Job drawing, mm, ordinate dimensions from the low corner. One solid piece. A direction names the side the tool comes from. Give positions to 0.01 mm unless a question says otherwise; leave off trailing zeros. Order: outer loops, then holes, each group sorted by start corner. A loop starts at its lowest first (then second) coordinate and runs counter-clockwise, first axis right, second up.
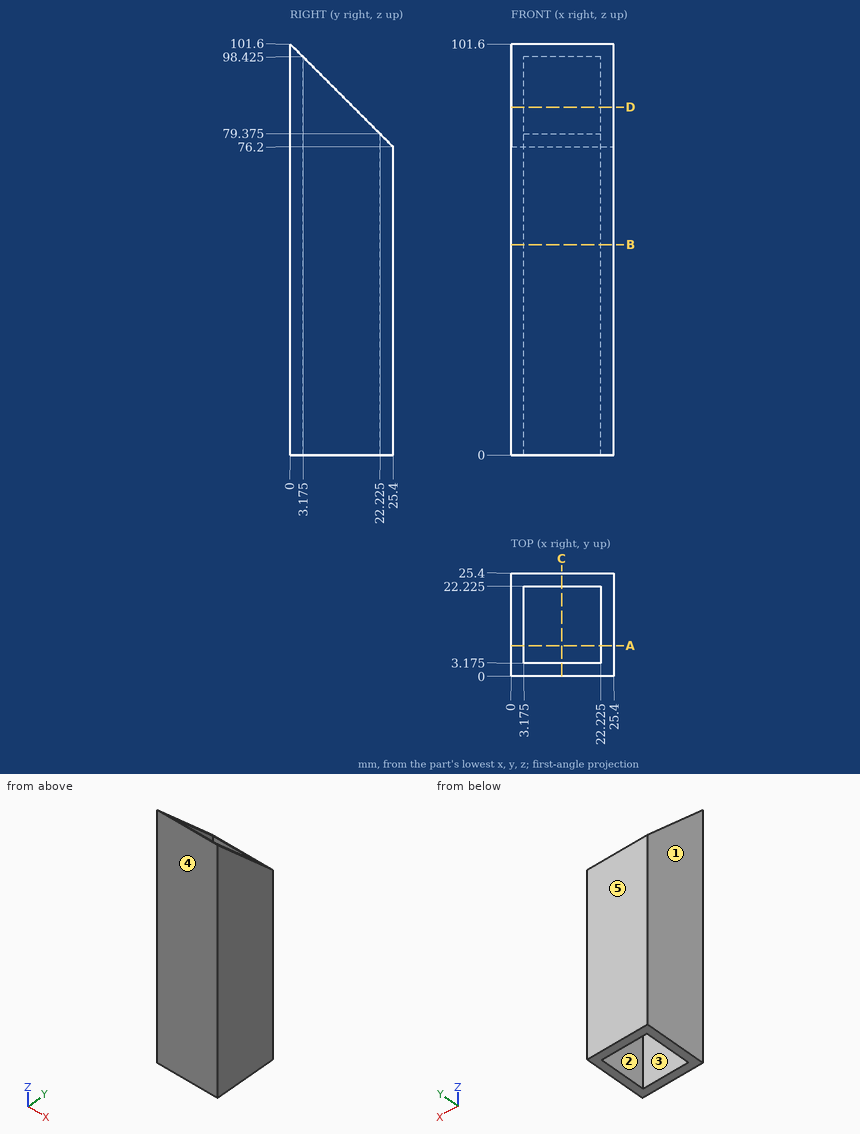
Item 1: Pull direction Y, two halves, no side cores. Call the marked faces 3, 4 and 5: released by +Y, released by -Y, zero draft, split by the parting line, or undercut.
Item 2: Band-saw the part on C-C on x = 12.5. List the corners of the cut face in (y, z) (3 decimals).
Item 3: Band-saw the part on A-A on y = 7.5. List the corners of the cut face in (x, z) (3 decimals), plus the area to 3 significant figures.
Item 4: Which spindle directions (+Z, -Z, +X, -X, +Y, -Y) get a long thin tool onto all of the face, cutting with end or side? Do the marked faces 1 and 2. Say none if no direction does.
Item 5: Band-saw the part on B-B on z = 52. List the corners of the cut face in (x, y) (3 decimals).
Item 6: Band-saw the part on D-D on z = 86. List the corners of the cut face in (x, y) (3 decimals).
Item 7: Drill centre lines: probe 1 along X at (y, z) = (18.25, 66.5) (3 decimals); probe 2 along Y at (x, z) = (20, 97) (3 decimals). Where is each one in solid material? Low to high.
Working result:
1. face 3: undercut
1. face 4: released by -Y
1. face 5: released by +Y
2. outline: (0, 0) - (3.175, 0) - (3.175, 98.425) - (0, 101.6) - close; (22.225, 0) - (25.4, 0) - (25.4, 76.2) - (22.225, 79.375) - close
3. outline: (0, 0) - (3.175, 0) - (3.175, 94.1) - (0, 94.1) - close; (22.225, 0) - (25.4, 0) - (25.4, 94.1) - (22.225, 94.1) - close
3. area: 598 mm2
4. face 1: +Z, -Z, -X, +Y, -Y
4. face 2: +Z, -Z
5. outline: (0, 0) - (25.4, 0) - (25.4, 25.4) - (0, 25.4) - close; hole (3.175, 3.175) - (22.225, 3.175) - (22.225, 22.225) - (3.175, 22.225) - close
6. outline: (0, 0) - (25.4, 0) - (25.4, 15.6) - (22.225, 15.6) - (22.225, 3.175) - (3.175, 3.175) - (3.175, 15.6) - (0, 15.6) - close
7. probe 1: x = 0 to 3.175, 22.225 to 25.4
7. probe 2: y = 0 to 3.175
